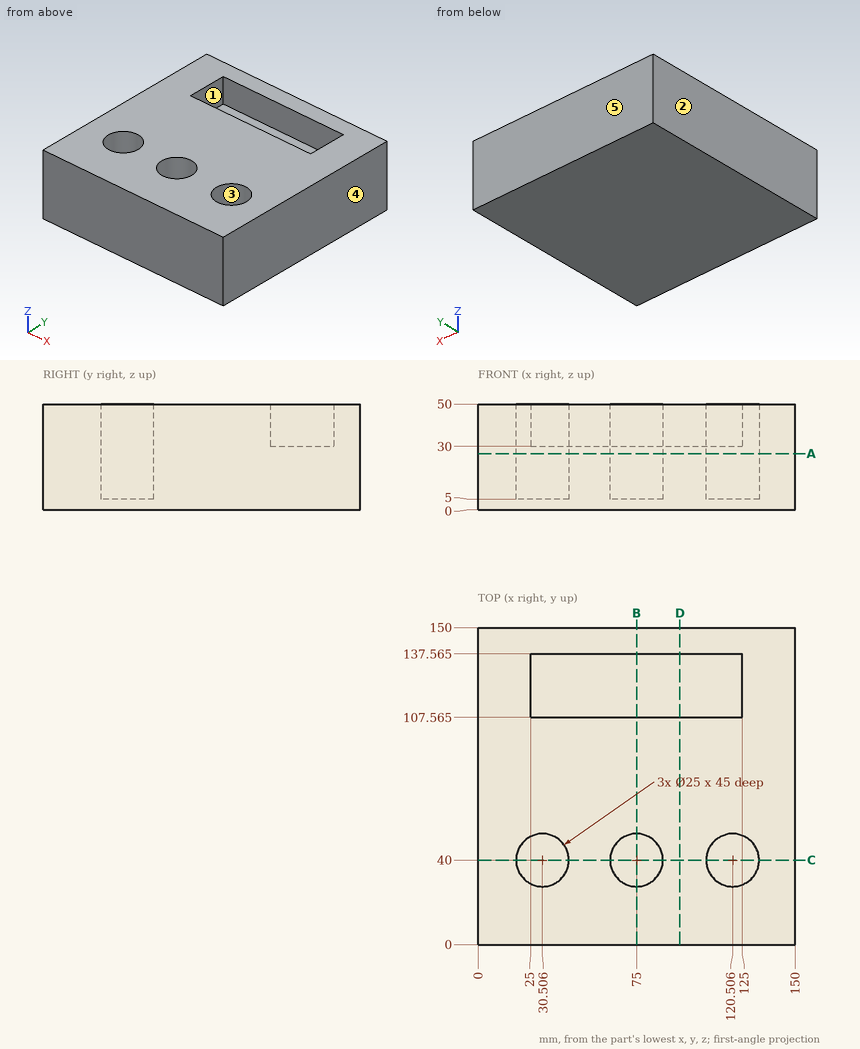
Study the drawing (mm; zero at the part's minimum x, y, z) and answer. A direction names the side the tool comes from. Give positions to 0.01 mm unless a question says otherwise; leave off trailing zeros. Write each loop counter-clockwise with the first axis right and the second up, starting at its lowest first coordinate (ties: lowest second). Pieces come first, ordered by that corner, then holes.
(1) The part is cut by section A-A on z = 26.5. Write down the section's boundary in (x, y), plus the area to 3 significant figures.
Final values:
outline: (0, 0) - (150, 0) - (150, 150) - (0, 150) - close; hole circle Ø25 at (30.51, 40); hole circle Ø25 at (75, 40); hole circle Ø25 at (120.51, 40)
area: 21,000 mm2
(2) A flat-ended cylindrical pin translates along its axis: pin 1 Ø7.5 at (x, y) = (35.5, 35.5) entering from +Z. Find the tip coordinate at first contact, or state that the pin passes through.
Final values:
pin 1: stops at z = 5
(3) Straight lines are drawn through the part: line 1 (Y direction, x = 75, z = 37) (3 decimals); line 2 (Y direction, x = 71.5, z = 46.5) (3 decimals); line 3 (Y direction, x = 128, z = 20) (1 decimal). For each, find the intervals that lie inside material, in ascending order.
Final values:
line 1: y = 0 to 27.5, 52.5 to 107.565, 137.565 to 150
line 2: y = 0 to 28, 52 to 107.565, 137.565 to 150
line 3: y = 0 to 30, 50 to 150
(4) The mould has two halves that part along X. Classify the marked faces 3, 4 and 5: pulls with the +X half, pulls with the -X half, needs draft (parallel to the pull), parting line crosses it, or undercut.
Final values:
face 3: undercut
face 4: pulls with the +X half
face 5: needs draft
(5) The part is cut by section D-D on x = 95.5. Write down the section's boundary in (y, z) (3 decimals), plus the area to 3 significant figures.
Final values:
outline: (0, 0) - (150, 0) - (150, 50) - (137.565, 50) - (137.565, 30) - (107.565, 30) - (107.565, 50) - (0, 50) - close
area: 6,900 mm2
(6) The part is cut by section C-C on y = 40. Write down the section's boundary in (x, z), plus the area to 4 significant figures.
Final values:
outline: (0, 0) - (150, 0) - (150, 50) - (133.01, 50) - (133.01, 5) - (108.01, 5) - (108.01, 50) - (87.5, 50) - (87.5, 5) - (62.5, 5) - (62.5, 50) - (43.01, 50) - (43.01, 5) - (18.01, 5) - (18.01, 50) - (0, 50) - close
area: 4,125 mm2
(7) The part is cut by section B-B on x = 75. Write down the section's boundary in (y, z) (3 decimals).
Final values:
outline: (0, 0) - (150, 0) - (150, 50) - (137.565, 50) - (137.565, 30) - (107.565, 30) - (107.565, 50) - (52.5, 50) - (52.5, 5) - (27.5, 5) - (27.5, 50) - (0, 50) - close
(8) Which of the six approach directions +Z, -Z, +X, -X, +Y, -Y give full straight-line access (tool end or side, diameter ignored) to the marked faces 1 and 2?
Final values:
face 1: +Z
face 2: +Z, -Z, -X, +Y, -Y
